Here's how the part is built. I have some questions about the finished solid (model axes, mm). A direction names the side the tool comes from. Coordinates: 2 decimals unless noted, no trailing zeros. Write each loop counter-clockwise with the first axis right and the second up, starting at its lowest first coordinate (ties: lowest second). Pieces come first, ordered by that corner, then holes. Notation, with made-up numbers: (-36.75, 8) -> (4.25, 8) arc R34 ccw to (4.25, 45) -> close; hole circle Ø1 at (23.25, 61). An arc over 180 degrees is marked (long way). Use a Markdown table: item, result. Add a question column.
```python
from build123d import *

# Parameters (mm, degrees)
EXTRUDE_1_DEPTH     = 4
SKETCH_2_R          = 4.25
EXTRUDE_2_DEPTH     = 1.9
SKETCH_3_R          = 3
CUT_EXTRUDE_1_DEPTH = 9.9


with BuildPart() as part:
    # 草图1 → 凸台-拉伸1 (new body)
    with BuildSketch(Plane.XY):
        Polygon((0, 5.773502692), (-5, 2.886751346), (-5, -2.886751346), (0, -5.773502692), (5, -2.886751346), (5, 2.886751346), align=None)
    extrude(amount=EXTRUDE_1_DEPTH)

    # 草图2 → 凸台-拉伸2 (add)
    with BuildSketch(Plane.XY.offset(4)):
        with Locations(Location((0, 0, 0), (0, 0, 180))):
            Circle(SKETCH_2_R)
    extrude(amount=EXTRUDE_2_DEPTH)

    # 草图3 → 切除-拉伸1 (cut)
    with BuildSketch(Plane.XY.offset(5.9)):
        Circle(SKETCH_3_R)
    extrude(amount=-CUT_EXTRUDE_1_DEPTH, mode=Mode.SUBTRACT)


solid = part.part
```
Q1. Thinking about a two-plate mould opening in Y: for faces 1 (the flat face through (-5, 0, 2)), 2 (the cylindrical face through (0.553, -4.214, 4.937)), 3 (the flat face through (-2.465, 4.35, 1.972)), 4 (the cylindrical face through (-3, 0, 3)), which applies, released by +Y, released by -Y, zero draft, split by the parting line, or undercut?
Q2. Suppose I cut it at A-A, the plane y = 0. Write out the boundary of the cut face in (x, z), and give its area (4 significant figures).
Q3. Which directions (+Z, -Z, +X, -X, +Y, -Y) give clear straight access to the entire face, cutting with the end or side of a thin tool? Please do faces 5 (the flat face through (5, 0, 2)), 6 (the flat face through (-2, -4, 4)).
Q4. Will these pins go through, and if not, where does the flat tip stop? pin 1 (1 mm diameter, centred on y = -4.5, z = 1.5, fed in from -X); pin 2 (1 mm diameter, centred on y = -3.5, z = 3, fed in from +X); pin 3 (3.5 mm diameter, centred on x = 0, y = 0, fed in from +Z).
Q5. Suppose I cut it at C-C, the plane x = 2.5. Write out the boundary of the cut face in (y, z), and give its area (3 significant figures).
Q6. Suppose I cut it at D-D, the plane x = 4. Write out the boundary of the cut face in (y, z), and give its area (3 significant figures).
Q7. Please list where these lines run through material, in increasing order: line 1 (Y direction, x = 0, z = 4.7); line 2 (Z direction, x = -0.75, y = 4.75); line 3 (X direction, y = 1, z = 3.5).
Q8. Suppose I cut it at B-B, the plane z = 2.7. Write out the boundary of the cut face in (x, y), and give its area (3 significant figures).
Answer key:
| question | item | result |
|---|---|---|
| 1 | face 1 | zero draft |
| 1 | face 2 | split by the parting line |
| 1 | face 3 | released by +Y |
| 1 | face 4 | undercut |
| 2 | outline | (-5, 0) -> (-3, 0) -> (-3, 5.9) -> (-4.25, 5.9) -> (-4.25, 4) -> (-5, 4) -> close; (3, 0) -> (5, 0) -> (5, 4) -> (4.25, 4) -> (4.25, 5.9) -> (3, 5.9) -> close |
| 2 | area | 20.75 mm^2 |
| 3 | face 5 | +Z, -Z, +X, +Y, -Y |
| 3 | face 6 | +Z |
| 4 | pin 1 | stops at x = -3.07 |
| 4 | pin 2 | stops at x = 4.8 |
| 4 | pin 3 | passes through |
| 5 | outline | (-4.33, 0) -> (-1.66, 0) -> (-1.66, 5.9) -> (-3.44, 5.9) -> (-3.44, 4) -> (-4.33, 4) -> close; (1.66, 0) -> (4.33, 0) -> (4.33, 4) -> (3.44, 4) -> (3.44, 5.9) -> (1.66, 5.9) -> close |
| 5 | area | 28.1 mm^2 |
| 6 | outline | (-3.46, 0) -> (3.46, 0) -> (3.46, 4) -> (1.44, 4) -> (1.44, 5.9) -> (-1.44, 5.9) -> (-1.44, 4) -> (-3.46, 4) -> close |
| 6 | area | 33.2 mm^2 |
| 7 | line 1 | y = -4.25 to -3, 3 to 4.25 |
| 7 | line 2 | z = 0 to 4 |
| 7 | line 3 | x = -5 to -2.83, 2.83 to 5 |
| 8 | outline | (-5, -2.89) -> (0, -5.77) -> (5, -2.89) -> (5, 2.89) -> (0, 5.77) -> (-5, 2.89) -> close; hole circle Ø6 at (0, 0) |
| 8 | area | 58.3 mm^2 |
